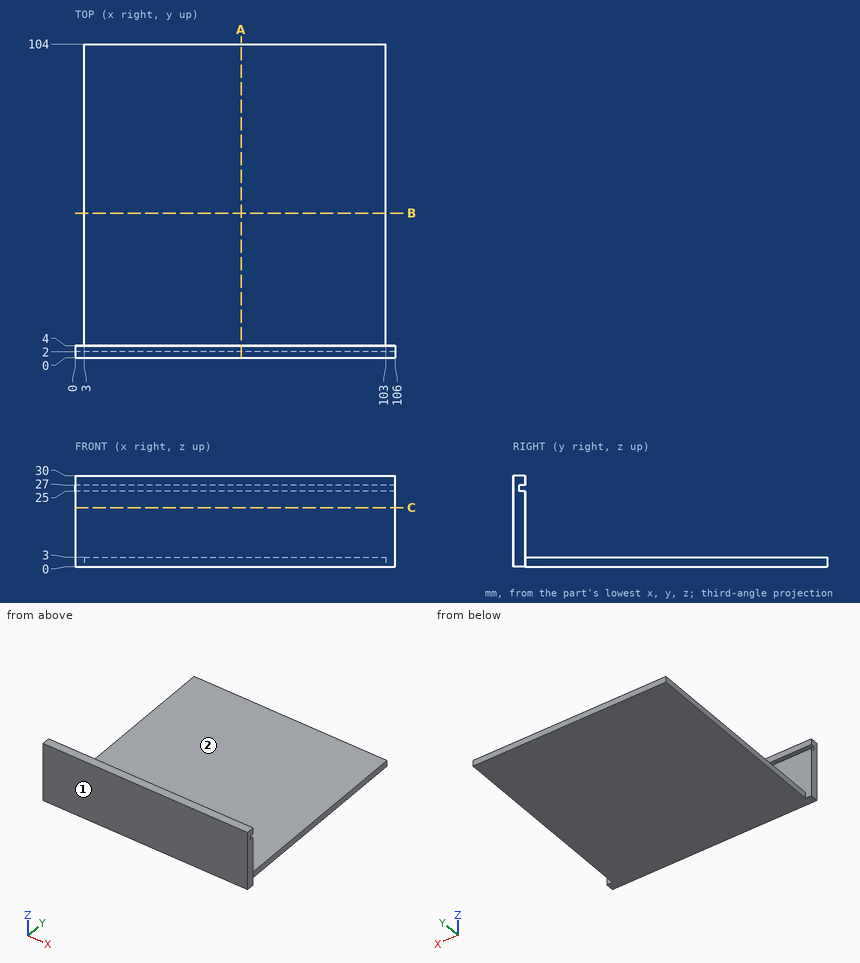
Geometry check sheet. Reference: drawing and pictorial views, mm from the part's lowest x, y, z. A direction names the side the tool comes from. Give positions to 0.01 mm unless a question says otherwise; leave off trailing zeros. Order: outer loops, then holes, each group sorted by start corner. A loop starts at its lowest first (then second) coordinate and runs counter-clockwise, first axis right, second up. Notation, with made-up numbers: M 63.5,65.25 L 89.5,65.25 A29 cw 89.5,90.25 Z; hole C -0.75,65 d9. An arc over 180 degrees is marked long. Return JSON: item names as keys, results as strings. Group by question number.
1) Scan lines: line 1 (Z direction, x = 35, y = 70.5); line 2 (Y direction, x = 37, z = 4.25); line 3 (Y direction, x = 49, z = 26.5). Record each from-to range of solid material in increasing order.
2) Access from +Z, -Z, +X, -X, +Y, -Y to the whole of each face (thin tool, end or side, straight path). Record for the marked faces 1 and 2.
3) Go/stop test with flat-tipped pins: pin 1 Ø7.5 at (x, z) = (69, 7.5) entering from +Y; pin 2 Ø1 at (x, y) = (22, 52.5) entering from +Z; pin 3 Ø1 at (x, y) = (53, 2.5) entering from -Z; pin 4 Ø0.9 at (y, z) = (66, 1.5) entering from +X. Record where each tip stops, or that it passes through.
4) Section check B-B on y = 48. Record the cut outline in (x, z), and give its area (3 significant figures).
5) Section check A-A on x = 55. Record the cut outline in (y, z), and give its area (3 significant figures).
6) Section check C-C on z = 19.5. Record the cut outline in (x, y).
Answer block:
{
 "1": {"line 1": "z = 0 to 3", "line 2": "y = 0 to 4", "line 3": "y = 0 to 2"},
 "2": {"face 1": "+Z, -Z, +X, -X, -Y", "face 2": "+Z, +X, -X, +Y"},
 "3": {"pin 1": "stops at y = 4", "pin 2": "stops at z = 3", "pin 3": "stops at z = 0", "pin 4": "stops at x = 103"},
 "4": {"outline": "M 3,0 L 103,0 L 103,3 L 3,3 Z", "area": "300 mm^2"},
 "5": {"outline": "M 0,0 L 104,0 L 104,3 L 4,3 L 4,25 L 2,25 L 2,27 L 4,27 L 4,30 L 0,30 Z", "area": "416 mm^2"},
 "6": {"outline": "M 0,0 L 106,0 L 106,4 L 0,4 Z"}
}
